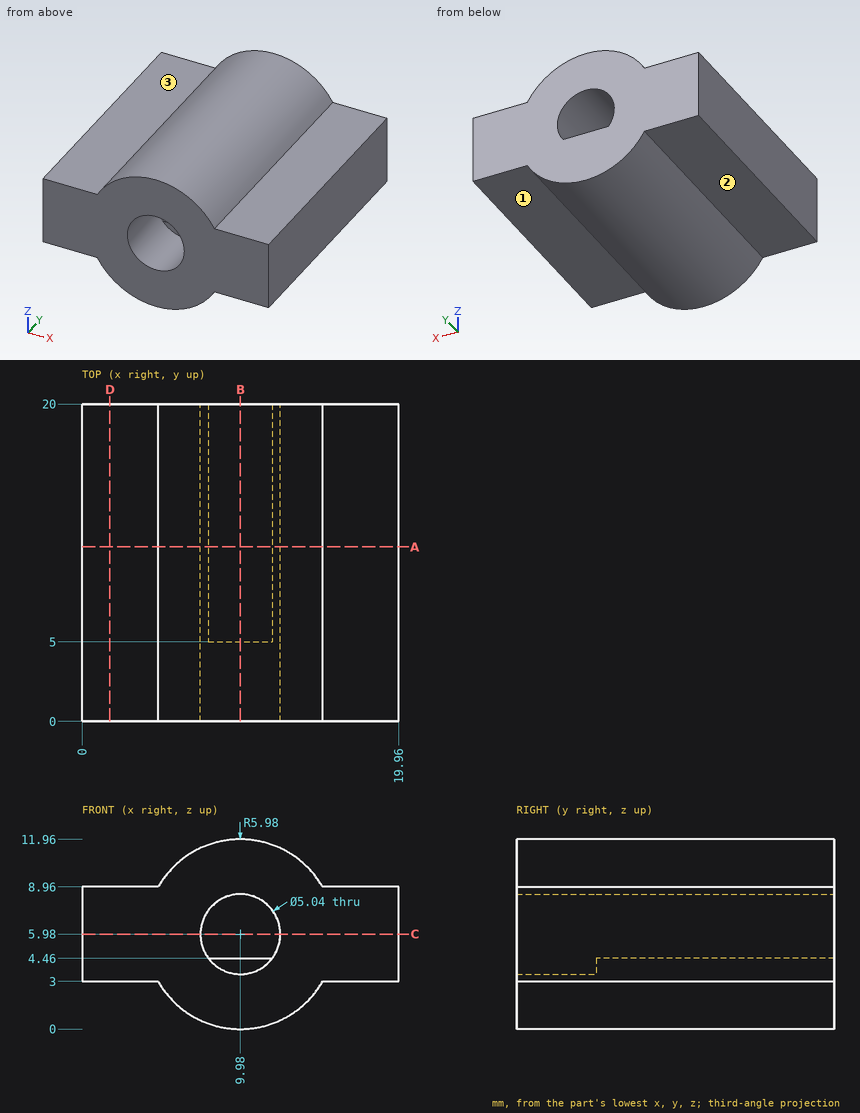
Study the drawing (mm; zero at the part's minimum x, y, z) and answer. A direction names the side the tool comes from. Coordinates: 2 decimals unless noted, no trailing zeros. Write each loop counter-clockwise with the first axis right and the second up, starting at its lowest first coordinate (ties: lowest second). Pieces come first, ordered by that corner, then holes. Notation, with made-up numbers: (-29.75, 34) - (-8.75, 34) arc R11 ccw to (-8.75, 49) - close; hole circle Ø3 at (72, -15). An arc over 180 degrees is marked (long way). Put each result on its own line as item: value.
1. The part is cut by section B-B on x = 9.98. Give the vertices of the cut face in (y, z).
Answer sheet:
outline: (0, 0) - (20, 0) - (20, 4.46) - (5, 4.46) - (5, 3.46) - (0, 3.46) - close; (0, 8.5) - (20, 8.5) - (20, 11.96) - (0, 11.96) - close
2. A tool of negligible diameter and unlimited length cuts with its end or side. For the marked faces 1, 2 and 3, from which of +Z, -Z, +X, -X, +Y, -Y can it reach the whole face along a straight path? Write none if from no direction.
Answer sheet:
face 1: -Z, +X, +Y, -Y
face 2: -Z, -X, +Y, -Y
face 3: +Z, -X, +Y, -Y
3. The part is cut by section C-C on z = 5.98. Give the vertices of the cut face in (x, y), plus the area to 3 significant figures.
Answer sheet:
outline: (0, 0) - (7.46, 0) - (7.46, 20) - (0, 20) - close; (12.5, 0) - (19.96, 0) - (19.96, 20) - (12.5, 20) - close
area: 298 mm^2
4. The part is cut by section A-A on y = 11. Give the vertices of the cut face in (x, z), plus the area to 3 significant figures.
Answer sheet:
outline: (0, 3) - (4.8, 3) arc R5.98 ccw to (15.16, 3) - (19.96, 3) - (19.96, 8.96) - (15.16, 8.96) arc R5.98 ccw to (4.8, 8.96) - (0, 8.96) - close; hole (7.97, 4.46) - (11.99, 4.46) arc R2.52 ccw (long way) to start
area: 146 mm^2
5. Find the intervals of material crossed by line 1 along X through (y, z) = (2.7, 5.98); line 2 along Z through (x, y) = (4.5, 3.25); line 3 along X through (y, z) = (7.5, 8), in increasing order. Write a range as from..to.
Answer sheet:
line 1: x = 0..7.46, 12.5..19.96
line 2: z = 3..8.96
line 3: x = 0..8.47, 11.49..19.96
6. The part is cut by section D-D on x = 1.75. Give the vertices of the cut face in (y, z), plus the area to 3 significant figures.
Answer sheet:
outline: (0, 3) - (20, 3) - (20, 8.96) - (0, 8.96) - close
area: 119 mm^2
7. Flat-ended cylindrical pins translate along their axes: pin 1 Ø1 at (x, y) = (13.5, 15) entering from -Z; pin 2 Ø10 at (x, y) = (6.5, 14.5) entering from -Z; pin 3 Ø4 at (x, y) = (1, 11) entering from -Z; pin 4 Ø1.4 at (x, y) = (1.5, 8.5) entering from +Z. Find the tip coordinate at first contact, or state that the pin passes through.
Answer sheet:
pin 1: stops at z = 0.82
pin 2: stops at z = 0
pin 3: stops at z = 3
pin 4: stops at z = 8.96
